Verification items for the finished model (mm, model axes). A direction names the side the tool comes from. Give positions to 0.01 mm unless a question says otherwise; leave off trailing zeros. Write each loop counter-clockwise with the first axis right and the second up, starting at its lowest first coordinate (ties: lowest second). Pieces come first, ordered by that corner, then holes. Notation, with made-up numbers: M -39.75,17.25 L -17.75,17.25 A22 ccw -17.75,34.25 Z; hole C 44.25,57.25 d8. An arc over 180 degrees is marked long. Write item = value, one per line.
from build123d import *

# Parameters (mm, degrees)
F0_R     = 2.667
F0_R_2   = 2.2479
F0_R_3   = 3.81
F1_DEPTH = 6.35
F2_R     = 20.32
F2_R_2   = 3.81
F3_DEPTH = 1.778
F4_SIZE  = 2.921


# Not quite as in the source:
# - a fillet or chamfer that OpenCascade refuses, or shapes differently, is made with other operations: its cross-section is extruded or revolved along the edge and cut away or added


with BuildPart() as f1:
    # F0 (on Front) → F1 (new body)
    with BuildSketch(Plane.XZ):
        with BuildLine():
            Line((-23.495, -28.575), (23.495, -28.575))
            ThreePointArc((23.495, -28.575), (27.0871024484, -27.0871024484), (28.575, -23.495))
            Line((28.575, -23.495), (28.575, -9.525))
            ThreePointArc((28.575, -9.525), (29.5049359697, -7.2799359697), (31.75, -6.35))
            Line((31.75, -6.35), (33.3375, -6.35))
            ThreePointArc((33.3375, -6.35), (39.6875, 0), (33.3375, 6.35))
            Line((33.3375, 6.35), (31.75, 6.35))
            ThreePointArc((31.75, 6.35), (29.5049359697, 7.2799359697), (28.575, 9.525))
            Line((28.575, 9.525), (28.575, 23.495))
            ThreePointArc((28.575, 23.495), (27.0871024484, 27.0871024484), (23.495, 28.575))
            Line((23.495, 28.575), (-23.495, 28.575))
            ThreePointArc((-23.495, 28.575), (-27.0871024484, 27.0871024484), (-28.575, 23.495))
            Line((-28.575, 23.495), (-28.575, 9.525))
            ThreePointArc((-28.575, 9.525), (-29.5049359697, 7.2799359697), (-31.75, 6.35))
            Line((-31.75, 6.35), (-33.3375, 6.35))
            ThreePointArc((-33.3375, 6.35), (-39.6875, 0), (-33.3375, -6.35))
            Line((-33.3375, -6.35), (-31.75, -6.35))
            ThreePointArc((-31.75, -6.35), (-29.5049359697, -7.2799359697), (-28.575, -9.525))
            Line((-28.575, -9.525), (-28.575, -23.495))
            ThreePointArc((-28.575, -23.495), (-27.0871024484, -27.0871024484), (-23.495, -28.575))
        make_face()
        with Locations((-23.495, -23.495)):
            Circle(F0_R, mode=Mode.SUBTRACT)
        with Locations((23.495, -23.495)):
            Circle(F0_R, mode=Mode.SUBTRACT)
        with Locations((-33.3375, 0)):
            Circle(F0_R_2, mode=Mode.SUBTRACT)
        with Locations((-23.495, 23.495)):
            Circle(F0_R, mode=Mode.SUBTRACT)
        Circle(F0_R_3, mode=Mode.SUBTRACT)
        with Locations((33.3375, 0)):
            Circle(F0_R_2, mode=Mode.SUBTRACT)
        with Locations((23.495, 23.495)):
            Circle(F0_R, mode=Mode.SUBTRACT)
    extrude(amount=F1_DEPTH)

    # F2 (on face) → F3 (cut)
    with BuildSketch(Plane.XZ.offset(6.35)):
        Circle(F2_R)
        Circle(F2_R_2, mode=Mode.SUBTRACT)
        Circle(F2_R)
    extrude(amount=-F3_DEPTH, mode=Mode.SUBTRACT)

    # F4
    f4_edges = [f1.edges().sort_by_distance(p)[0] for p in [
        (-35.5854, -6.35, 0),
        (31.0896, -6.35, 0),
    ]]
    chamfer(f4_edges, length=F4_SIZE)

    # F5: chamfer of 3.429 on 4 edges, made by hand

    # F5_s1 → F5_t2 (revolve, cut)
    with BuildSketch(Plane.XY.offset(23.495)):
        Polygon((26.162, -3.429), (29.591, 0), (26.162, 0), align=None)
    revolve(axis=Axis((23.495, 0, 23.495), (0, -1, 0)), mode=Mode.SUBTRACT)

    # F5_s3 → F5_t4 (revolve, cut)
    with BuildSketch(Plane.XY.offset(23.495)):
        Polygon((-20.828, -3.429), (-17.399, 0), (-20.828, 0), align=None)
    revolve(axis=Axis((-23.495, 0, 23.495), (0, -1, 0)), mode=Mode.SUBTRACT)

    # F5_s5 → F5_t6 (revolve, cut)
    with BuildSketch(Plane.XY.offset(-23.495)):
        Polygon((26.162, -3.429), (29.591, 0), (26.162, 0), align=None)
    revolve(axis=Axis((23.495, 0, -23.495), (0, -1, 0)), mode=Mode.SUBTRACT)

    # F5_s7 → F5_t8 (revolve, cut)
    with BuildSketch(Plane.XY.offset(-23.495)):
        Polygon((-20.828, -3.429), (-17.399, 0), (-20.828, 0), align=None)
    revolve(axis=Axis((-23.495, 0, -23.495), (0, -1, 0)), mode=Mode.SUBTRACT)


solid = f1.part
1) Cross-section at C-C on y = -2.5. Count the separate pieces of the cut face and the enclosed holes in it, plus the area to 3 significant figures.
From the geometry:
separate_pieces = 1
enclosed_holes = 7
area = 3,260 mm^2
2) Cross-section at A-A on x = 0. Record the boundary of the cut face in (y, z) (3 decimals).
From the geometry:
outline = M -6.35,-28.575 L 0,-28.575 L 0,-3.81 L -4.572,-3.81 L -4.572,-20.32 L -6.35,-20.32 Z; M -6.35,20.32 L -4.572,20.32 L -4.572,3.81 L 0,3.81 L 0,28.575 L -6.35,28.575 Z
3) Depth check by flat-ended pin: P1, Ø24.5, axis at x = 0, z = 0, coming from the -Y side; P2, Ø1.9, axis at y = -4.5, z = 19, coming from the +X side (3 decimals); P3, Ø1.5, axis at x = -26.5, y = -1.5, coming from the +Z side; P4, Ø3, axis at x = 23.495, z = -23.495, coming from the -Y side. Enter the tip coordinate at first touch or a pass-through.
From the geometry:
P1 = -4.57
P2 = 28.575
P3 = 28.05
P4 = through
4) Cross-section at B-B on z = 0. Record the boundary of the cut face in (x, y).
From the geometry:
outline = M -39.69,-6.35 L -38.51,-6.35 L -35.59,-3.43 L -35.59,0 L -39.69,0 Z; M -31.09,-3.43 L -28.17,-6.35 L -20.32,-6.35 L -20.32,-4.57 L -3.81,-4.57 L -3.81,0 L -31.09,0 Z; M 3.81,-4.57 L 20.32,-4.57 L 20.32,-6.35 L 28.17,-6.35 L 31.09,-3.43 L 31.09,0 L 3.81,0 Z; M 35.59,-3.43 L 38.51,-6.35 L 39.69,-6.35 L 39.69,0 L 35.59,0 Z
5) Tool access check on faces 4 (the flat face through (-28.575, -3, -16)), 5 (the cylindrical face through (35.414, -1.69, -0.861)), 6 (the flat face through (33, -3, 6.35)). Record the directions out of +Z, -Z, +X, -X, +Y, -Y that give a thin tool (end or side, any length) a straight path to the whole face; none if there is none.
From the geometry:
face_4 = -Z, -X, +Y, -Y
face_5 = +Y, -Y
face_6 = +Z, +X, +Y, -Y
6) Material ranges on probe 1 along X at (y, z) = (-5, 23.5) (3 decimals); probe 2 along Z at (x, y) = (-19.5, -0.75) (3 decimals); probe 3 along Y at (x, z) = (-16.5, 11.5), recorded low to high. Write a range as from..to.
From the geometry:
probe_1 = -28.575..-26.162, -20.828..20.828, 26.162..28.575
probe_2 = -28.575..-27.047, -19.943..19.943, 27.047..28.575
probe_3 = -4.57..0
7) Draft check along X on faces 1 (the cylindrical face through (29.53, -3.131, 7.255)), 2 (the flat face through (-33, -3, 6.35)), 3 (the conical face through (-21.946, -3.214, -21.065)). Enter one of: +X half, -X half, draft (parallel to the pull), parting line (faces both ways), or undercut.
From the geometry:
face_1 = +X half
face_2 = draft
face_3 = undercut
